Work out the finished part from the listing and answer in its coordinate system (mm). A direction names the side the tool comes from. Coordinates: 2 decimals unless noted, no trailing zeros. Write each loop counter-clockwise with the first axis right and the second up, starting at its lowest first coordinate (ties: lowest second). Pieces come first, ordered by that corner, then holes. Notation, with made-up numbers: (83, 81.25) - (87, 81.25) arc R28 ccw to (87, 102.25) - close; hole circle Ø11 at (51.25, 62). An arc over 180 degrees is marked (long way). Use a Markdown table: item, result. Add a question column.
(1) The part is cut by section D-D, the plane z = -1.35. Give the vertices of the cut face in (x, y), then the cut area to 3 significant figures.
(2) Find the intervals of material crossed by line 1 (X direction, y = 8, z = 0); line 2 (X direction, y = 7, z = 1); line 3 (Z direction, x = 0.8, y = 1.25), in increasing order. Write a range as from..to.
(3) Given pin 1 Ø1.4 at (y, z) = (8.5, -1.5) entering from -X; pin 2 Ø0.5 at (x, z) = (0, -2) entering from +Y; pin 3 Ø0.7 at (y, z) = (8, -1.5) entering from +X, each flat-ended and moving along its own axis, determine where each tip first touches the part or whether it passes through.
(4) For a pull along Z with two mould halves and no side action, classify faces 3 (the face through (0, 6, -2)), 4 (the face through (0.08, 5.92, 1.8)), 5 (the face through (-1.05, 5.92, 2.54)) as released by +Z, released by -Z, zero draft, split by the parting line, or undercut.
(5) The part is cut by section A-A, the plane x = 0. Give the vertices of the cut face in (y, z), then the cut area to 3 significant figures.
(6) The part is cut by section C-C, the plane y = 4.25. Give the vertices of the cut face in (x, z).
(7) A tool of negligible diameter and unlimited length cuts with its end or side. For faces 1 (the face through (0, 12, 2)), 2 (the face through (-1.5, 9, -2)), from which of +Z, -Z, +X, -X, +Y, -Y can it reach the whole face along a straight path? Write none if from no direction.
(8) The part is cut by section B-B, the plane z = 0. Give the vertices of the cut face in (x, y), then the cut area to 3 significant figures.
from build123d import *

# Parameters (mm, degrees)
SKETCH1_R           = 2.75
BOSS_EXTRUDE1_DEPTH = 12
SKETCH3_R           = 1.8
CUT_EXTRUDE1_DEPTH  = 12
SKETCH4_W           = 3
SKETCH4_H           = 2.75
CUT_EXTRUDE2_DEPTH  = 6


with BuildPart() as part:
    # Sketch1 → Boss-Extrude1 (new body)
    with BuildSketch(Plane(origin=(0, 0, 0), x_dir=(1, 0, 0), z_dir=(0, 1, 0))):
        with Locations(Location((0, 0, 0), (0, 0, 270))):
            Circle(SKETCH1_R)
    extrude(amount=BOSS_EXTRUDE1_DEPTH)

    # Sketch3 → Cut-Extrude1 (cut)
    with BuildSketch(Plane.XZ):
        with Locations(Location((0, 0, 0), (0, 0, 270))):
            Circle(SKETCH3_R)
    extrude(amount=-CUT_EXTRUDE1_DEPTH, mode=Mode.SUBTRACT)

    # Sketch4 → Cut-Extrude2 (cut)
    with BuildSketch(Plane(origin=(0, 12, 0), x_dir=(1, 0, 0), z_dir=(0, 1, 0))):
        with Locations((0, 1.375)):
            Rectangle(SKETCH4_W, SKETCH4_H)
    extrude(amount=-CUT_EXTRUDE2_DEPTH, mode=Mode.SUBTRACT)


solid = part.part
Model answer:
| question | item | result |
|---|---|---|
| 1 | outline | (-2.4, 0) - (-1.19, 0) - (-1.19, 6) - (-1.5, 6) - (-1.5, 12) - (-2.4, 12) - close; (1.19, 0) - (2.4, 0) - (2.4, 12) - (1.5, 12) - (1.5, 6) - (1.19, 6) - close |
| 1 | area | 25.2 mm^2 |
| 2 | line 1 | -2.75..-1.8, 1.8..2.75 |
| 2 | line 2 | -2.56..-1.5, 1.5..2.56 |
| 2 | line 3 | -2.63..-1.61, 1.61..2.63 |
| 3 | pin 1 | x = -2.63 |
| 3 | pin 2 | y = 6 |
| 3 | pin 3 | x = 2.5 |
| 4 | face 3 | zero draft |
| 4 | face 4 | undercut |
| 4 | face 5 | split by the parting line |
| 5 | outline | (0, -2.75) - (6, -2.75) - (6, -1.8) - (0, -1.8) - close; (0, 1.8) - (12, 1.8) - (12, 2.75) - (0, 2.75) - close |
| 5 | area | 17.1 mm^2 |
| 6 | outline | circle Ø5.5 at (0, 0); hole circle Ø3.6 at (0, 0) |
| 7 | face 1 | +Z, -Z, +X, -X, +Y |
| 7 | face 2 | -Z, +Y |
| 8 | outline | (-2.75, 0) - (-1.8, 0) - (-1.8, 12) - (-2.75, 12) - close; (1.8, 0) - (2.75, 0) - (2.75, 12) - (1.8, 12) - close |
| 8 | area | 22.8 mm^2 |
